```python
from build123d import *

# Parameters (mm, degrees)
SKETCH_4_R       = 5
EXTRUDE_4_DEPTH  = 57
SKETCH_5_R       = 3.5
EXTRUDE_5_DEPTH  = 2
EXTRUDE_START    = 12
SKETCH_6_R       = 5
EXTRUDE_6_DEPTH  = 12
EXTRUDE_START_2  = 2
SKETCH_7_R       = 3.5
EXTRUDE_7_DEPTH  = 2
SKETCH_8_R       = 5
EXTRUDE_8_DEPTH  = 12
SKETCH_9_R       = 3.5
EXTRUDE_9_DEPTH  = 2
SKETCH_10_R      = 5
EXTRUDE_10_DEPTH = 3
SKETCH_11_R      = 3.5
EXTRUDE_11_DEPTH = 2
SKETCH_12_R      = 5
EXTRUDE_12_DEPTH = 24
SKETCH_13_R      = 3.5
EXTRUDE_13_DEPTH = 2
SKETCH_14_R      = 5
EXTRUDE_14_DEPTH = 25
SKETCH_15_R      = 3.5
EXTRUDE_15_DEPTH = 2
SKETCH_16_R      = 5
EXTRUDE_16_DEPTH = 10
SKETCH_33_R      = 3.5
EXTRUDE_25_DEPTH = 2
EXTRUDE_START_3  = 3
SKETCH_34_R      = 5
EXTRUDE_26_DEPTH = 3
SKETCH_35_R      = 3.5
EXTRUDE_27_DEPTH = 2
EXTRUDE_START_4  = 24
SKETCH_36_R      = 5
EXTRUDE_28_DEPTH = 24
SKETCH_37_R      = 3.5
EXTRUDE_29_DEPTH = 2
EXTRUDE_START_5  = 25
SKETCH_38_R      = 5
EXTRUDE_30_DEPTH = 25
SKETCH_39_R      = 3.5
EXTRUDE_31_DEPTH = 2
EXTRUDE_START_6  = 10
SKETCH_40_R      = 5
EXTRUDE_32_DEPTH = 10
CHAMFER_1_SIZE   = 0.5


with BuildPart() as part:
    # 草图4 → 凸台-拉伸4 (new body)
    with BuildSketch(Plane(origin=(0, 0, 0), x_dir=(0, 0, -1), z_dir=(1, 0, 0))):
        with Locations(Location((0, 0, 0), (0, 0, 180))):
            Circle(SKETCH_4_R)
    extrude(amount=EXTRUDE_4_DEPTH)

    # 草图5 → 凸台-拉伸5 (add)
    with BuildSketch(Plane.ZY):
        Circle(SKETCH_5_R)
    extrude(amount=EXTRUDE_5_DEPTH)

    # 草图6 → 凸台-拉伸6 (add)
    with BuildSketch(Plane.ZY.offset(2).offset(EXTRUDE_START)):
        Circle(SKETCH_6_R)
    extrude(amount=-EXTRUDE_6_DEPTH)

    # 草图7 → 凸台-拉伸7 (add)
    with BuildSketch(Plane(origin=(57, 0, 0), x_dir=(0, 0, -1), z_dir=(1, 0, 0)).offset(EXTRUDE_START_2)):
        with Locations(Location((0, 0, 0), (0, 0, 180))):
            Circle(SKETCH_7_R)
    extrude(amount=-EXTRUDE_7_DEPTH)

    # 草图8 → 凸台-拉伸8 (add)
    with BuildSketch(Plane(origin=(59, 0, 0), x_dir=(0, 0, -1), z_dir=(1, 0, 0))):
        with Locations(Location((0, 0, 0), (0, 0, 180))):
            Circle(SKETCH_8_R)
    extrude(amount=EXTRUDE_8_DEPTH)

    # 草图9 → 凸台-拉伸9 (add)
    with BuildSketch(Plane(origin=(71, 0, 0), x_dir=(0, 0, -1), z_dir=(1, 0, 0)).offset(EXTRUDE_START_2)):
        with Locations(Location((0, 0, 0), (0, 0, 180))):
            Circle(SKETCH_9_R)
    extrude(amount=-EXTRUDE_9_DEPTH)

    # 草图10 → 凸台-拉伸10 (add)
    with BuildSketch(Plane(origin=(73, 0, 0), x_dir=(0, 0, -1), z_dir=(1, 0, 0))):
        with Locations(Location((0, 0, 0), (0, 0, 180))):
            Circle(SKETCH_10_R)
    extrude(amount=EXTRUDE_10_DEPTH)

    # 草图11 → 凸台-拉伸11 (add)
    with BuildSketch(Plane(origin=(76, 0, 0), x_dir=(0, 0, -1), z_dir=(1, 0, 0)).offset(EXTRUDE_START_2)):
        with Locations(Location((0, 0, 0), (0, 0, 180))):
            Circle(SKETCH_11_R)
    extrude(amount=-EXTRUDE_11_DEPTH)

    # 草图12 → 凸台-拉伸12 (add)
    with BuildSketch(Plane(origin=(78, 0, 0), x_dir=(0, 0, -1), z_dir=(1, 0, 0))):
        with Locations(Location((0, 0, 0), (0, 0, 180))):
            Circle(SKETCH_12_R)
    extrude(amount=EXTRUDE_12_DEPTH)

    # 草图13 → 凸台-拉伸13 (add)
    with BuildSketch(Plane(origin=(102, 0, 0), x_dir=(0, 0, -1), z_dir=(1, 0, 0)).offset(EXTRUDE_START_2)):
        with Locations(Location((0, 0, 0), (0, 0, 180))):
            Circle(SKETCH_13_R)
    extrude(amount=-EXTRUDE_13_DEPTH)

    # 草图14 → 凸台-拉伸14 (add)
    with BuildSketch(Plane(origin=(104, 0, 0), x_dir=(0, 0, -1), z_dir=(1, 0, 0))):
        with Locations(Location((0, 0, 0), (0, 0, 180))):
            Circle(SKETCH_14_R)
    extrude(amount=EXTRUDE_14_DEPTH)

    # 草图15 → 凸台-拉伸15 (add)
    with BuildSketch(Plane(origin=(129, 0, 0), x_dir=(0, 0, -1), z_dir=(1, 0, 0)).offset(EXTRUDE_START_2)):
        with Locations(Location((0, 0, 0), (0, 0, 180))):
            Circle(SKETCH_15_R)
    extrude(amount=-EXTRUDE_15_DEPTH)

    # 草图16 → 凸台-拉伸16 (add)
    with BuildSketch(Plane(origin=(131, 0, 0), x_dir=(0, 0, -1), z_dir=(1, 0, 0))):
        with Locations(Location((0, 0, 0), (0, 0, 180))):
            Circle(SKETCH_16_R)
    extrude(amount=EXTRUDE_16_DEPTH)

    # 草图33 → 凸台-拉伸25 (add)
    with BuildSketch(Plane.ZY.offset(14)):
        Circle(SKETCH_33_R)
    extrude(amount=EXTRUDE_25_DEPTH)

    # 草图34 → 凸台-拉伸26 (add)
    with BuildSketch(Plane.ZY.offset(16).offset(EXTRUDE_START_3)):
        Circle(SKETCH_34_R)
    extrude(amount=-EXTRUDE_26_DEPTH)

    # 草图35 → 凸台-拉伸27 (add)
    with BuildSketch(Plane.ZY.offset(19)):
        Circle(SKETCH_35_R)
    extrude(amount=EXTRUDE_27_DEPTH)

    # 草图36 → 凸台-拉伸28 (add)
    with BuildSketch(Plane.ZY.offset(21).offset(EXTRUDE_START_4)):
        Circle(SKETCH_36_R)
    extrude(amount=-EXTRUDE_28_DEPTH)

    # 草图37 → 凸台-拉伸29 (add)
    with BuildSketch(Plane.ZY.offset(45)):
        Circle(SKETCH_37_R)
    extrude(amount=EXTRUDE_29_DEPTH)

    # 草图38 → 凸台-拉伸30 (add)
    with BuildSketch(Plane.ZY.offset(47).offset(EXTRUDE_START_5)):
        Circle(SKETCH_38_R)
    extrude(amount=-EXTRUDE_30_DEPTH)

    # 草图39 → 凸台-拉伸31 (add)
    with BuildSketch(Plane.ZY.offset(72)):
        Circle(SKETCH_39_R)
    extrude(amount=EXTRUDE_31_DEPTH)

    # 草图40 → 凸台-拉伸32 (add)
    with BuildSketch(Plane.ZY.offset(74).offset(EXTRUDE_START_6)):
        Circle(SKETCH_40_R)
    extrude(amount=-EXTRUDE_32_DEPTH)

    # 倒角1
    chamfer_1_edges = [part.edges().sort_by_distance(p)[0] for p in [
        (141, 0, -5),
        (-84, 0, -5),
    ]]
    chamfer(chamfer_1_edges, length=CHAMFER_1_SIZE)


solid = part.part
```
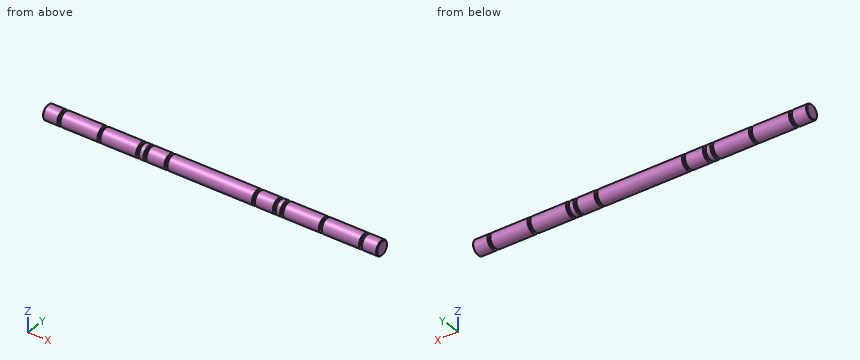
Verification items for the finished model (mm, model axes). Coordinates: 2 decimals unless noted, no trailing zeros. Loops run counter-clockwise (first coordinate to the right, second up) from the corner with the lowest first, then second, coordinate; pieces in that order, holes last. Notation, with made-up numbers: (43.5, 15.25) - (69.5, 15.25) arc R15 cw to (69.5, 23.25) - close; hole circle Ø2 at (4.5, -32.5). An arc over 180 degrees is marked (long way). Put each result on its own line as item: value.
Item 1: Gauge pin test, flat end, axial feed: pin 1 Ø6 at (x, z) = (58, 2.5) entering from +Y. Record the tip position at first contact, or that the pin passes through.
Conclusion:
pin 1: stops at y = 5
Item 2: Section check A-A (x = 31). Enter the section's corners in (y, z), then the cut area to 3 significant figures.
Conclusion:
outline: circle Ø10 at (0, 0)
area: 78.5 mm2
Item 3: Scan lines: line 1 along Z through (x, y) = (47, 0.25); line 2 along Y through (x, z) = (115.5, 0.5); line 3 along Y through (x, z) = (105.5, 2.25). Record each from-to range of solid material in increasing order.
Conclusion:
line 1: z = -4.99 to 4.99
line 2: y = -4.97 to 4.97
line 3: y = -4.47 to 4.47
